from build123d import *

# Parameters (mm, degrees)
SKETCH_1_R      = 1
EXTRUDE_1_DEPTH = 1.6
SKETCH_2_W      = 1.777379574
SKETCH_2_H      = 3.627987188
EXTRUDE_2_DEPTH = 1.7
SKETCH_3_W      = 4
SKETCH_3_H      = 10
SKETCH_3_W_2    = 10
SKETCH_3_H_2    = 4
EXTRUDE_3_DEPTH = 2


with BuildPart() as part:
    # 草图1 → 凸台-拉伸1 (new body)
    with BuildSketch(Plane.XY):
        with BuildLine():
            Line((-9.541571686, 14.6685), (9.591443257, 14.6685))
            ThreePointArc((9.591443257, 14.6685), (17.526, 0), (9.591443257, -14.6685))
            Line((9.591443257, -14.6685), (-9.541571686, -14.6685))
            ThreePointArc((-9.541571686, -14.6685), (-17.526, 0), (-9.541571686, 14.6685))
        make_face()
        with Locations((7.498513861, -7.498513861)):
            Circle(SKETCH_1_R, mode=Mode.SUBTRACT)
        with Locations((-7.498513861, 7.498513861)):
            Circle(SKETCH_1_R, mode=Mode.SUBTRACT)
        with Locations((7.498513861, 7.498513861)):
            Circle(SKETCH_1_R, mode=Mode.SUBTRACT)
    extrude(amount=EXTRUDE_1_DEPTH)

    # 草图2 → 凸台-拉伸2 (add)
    with BuildSketch(Plane(origin=(0, 0, 0), x_dir=(-1, 0, 0), z_dir=(0, 0, -1))):
        Rectangle(SKETCH_2_W, SKETCH_2_H)
    extrude(amount=EXTRUDE_2_DEPTH)

    # 草图3 → 凸台-拉伸3 (add)
    with BuildSketch(Plane.XY.offset(1.6)):
        with Locations((-12.555549106, 0)):
            Rectangle(SKETCH_3_W, SKETCH_3_H)
        with Locations((0, -12.555549106)):
            Rectangle(SKETCH_3_W_2, SKETCH_3_H_2)
        with Locations((0, 12.555549106)):
            Rectangle(SKETCH_3_W_2, SKETCH_3_H_2)
    extrude(amount=EXTRUDE_3_DEPTH)


solid = part.part
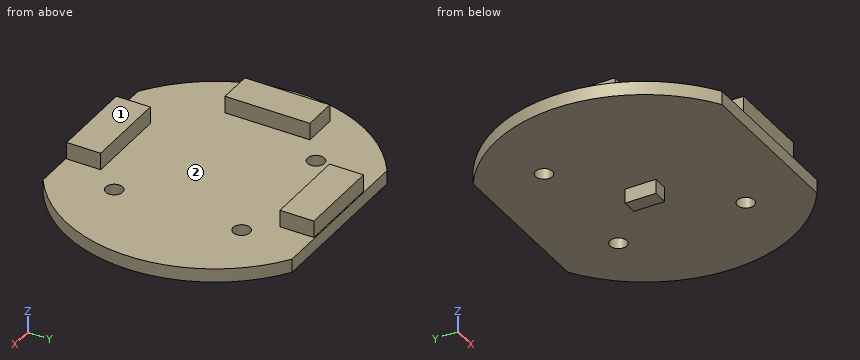
Work out the finished part from the listing and answer in its coordinate system (mm). Face numbers are marked on the shaded views. Round coordinates to 2 decimals unless told otherwise and drop trailing zeros. Loops run counter-clockwise (first coordinate to the right, second up) from the corner with the lowest first, then second, coordinate; pieces in that order, holes last. Notation, with made-up numbers: (-3.75, 53.25) - (6.25, 53.25) arc R19 ccw to (6.25, 84.25) - close; hole circle Ø3 at (-16.5, 49). An arc over 180 degrees is marked (long way). Use one line per item in the form item = value. Start each with the question number.
(1) Find section C-C on z = 0.85. Determine the outline of the cut face in (x, y), and give its area (3 significant figures).
(2) Find section B-B on x = -2. Determine the outline of the cut face in (y, z).
(3) Find section D-D on y = -2.5. Determine the outline of the cut face in (x, z).
(4) Determine the mould class of the marked faces 1 and 2 for opening direction Y: +Y half, -Y half, draft (parallel to the pull), parting line (faces both ways), or undercut.
(5) Consider line 1 (Z direction, x = 14, y = -2.5); line 2 (X direction, y = 10.75, z = 2.4); line 3 (Y direction, x = 0, z = -0.4). Determine where each line is inside the solid, lowest interval first.
(6) Flat-ended cylindrical pins translate along their axes: P1, Ø0.5, axis at y = 0.5, z = -0.5, coming from the -X side; P2, Ø3, axis at x = 13, z = -0.5, coming from the +Y side; P3, Ø0.6, axis at x = 0.5, z = 2.5, coming from the -Y side; P4, Ø1.8, axis at x = 7.5, y = -7.5, coming from the -Z side. Find the tip coordinate at first contact, or state that the pin passes through.
(7) Find section A-A on y = 8. Determine the outline of the cut face in (x, z), and give its area (3 significant figures).
Answer list:
q1.outline = (-9.54, -14.67) - (9.59, -14.67) arc R17.53 ccw to (9.59, 14.67) - (-9.54, 14.67) arc R17.47 ccw to start; hole circle Ø2 at (-7.5, 7.5); hole circle Ø2 at (7.5, -7.5); hole circle Ø2 at (7.5, 7.5)
q1.area = 881 mm^2
q2.outline = (-14.67, 0) - (14.67, 0) - (14.67, 1.6) - (14.56, 1.6) - (14.56, 3.6) - (10.56, 3.6) - (10.56, 1.6) - (-10.56, 1.6) - (-10.56, 3.6) - (-14.56, 3.6) - (-14.56, 1.6) - (-14.67, 1.6) - close
q3.outline = (-17.35, 0) - (17.35, 0) - (17.35, 1.6) - (-10.56, 1.6) - (-10.56, 3.6) - (-14.56, 3.6) - (-14.56, 1.6) - (-17.35, 1.6) - close
q4.face_1 = draft
q4.face_2 = undercut
q5.line_1 = 0 to 1.6
q5.line_2 = -5 to 5
q5.line_3 = -1.81 to 1.81
q6.P1 = -0.89
q6.P2 = 13.15
q6.P3 = -14.56
q6.P4 = through
q7.outline = (-15.59, 0) - (-8.36, 0) - (-8.36, 1.6) - (-15.59, 1.6) - close; (-6.63, 0) - (6.63, 0) - (6.63, 1.6) - (-6.63, 1.6) - close; (8.36, 0) - (15.59, 0) - (15.59, 1.6) - (8.36, 1.6) - close
q7.area = 44.4 mm^2
